from build123d import *

# Parameters (mm, degrees)
BOSS_EXTRUDE1_DEPTH = 4
SKETCH2_R           = 1.55
CUT_EXTRUDE3_DEPTH  = 130.223312929
FILLET1_R           = 5
SKETCH5_R           = 1.525
CUT_EXTRUDE4_DEPTH  = 10
SKETCH5_3_R         = 4.5
CUT_EXTRUDE5_DEPTH  = 1
CUT_EXTRUDE6_DEPTH  = 2.4
SKETCH8_W           = 140
SKETCH8_H           = 25
BOSS_EXTRUDE4_DEPTH = 5
CUT_EXTRUDE7_DEPTH  = 186.792392805
FILLET5_R           = 5
SKETCH12_W          = 5.5
SKETCH12_H          = 5
CUT_EXTRUDE8_DEPTH  = 10
FILLET6_R           = 1


with BuildPart() as part:
    # Sketch1 → Boss-Extrude1 (new body)
    with BuildSketch(Plane(origin=(0, 0, 0), x_dir=(1, 0, 0), z_dir=(0, 1, 0))):
        Polygon((-94.307015775, 45.137931034), (-94.307015775, 16.137931034), (-114.307015775, 16.137931034), (-114.307015775, 1.137931034), (-68.307015775, 1.137931034), (45.692984225, 1.137931034), (65.692984225, 1.137931034), (65.692984225, 16.137931034), (45.692984225, 16.137931034), (45.692984225, 45.137931034), (65.692984225, 45.137931034), (65.692984225, 60.137931034), (45.692984225, 60.137931034), (-68.307015775, 60.137931034), (-114.307015775, 60.137931034), (-114.307015775, 45.137931034), align=None)
    extrude(amount=BOSS_EXTRUDE1_DEPTH)

    # Sketch2 → Cut-Extrude3 (cut, through all)
    with BuildSketch(Plane(origin=(0, 4, 0), x_dir=(1, 0, 0), z_dir=(0, 1, 0))):
        with Locations(Location((40.192984225, 53.637931034, 0), (0, 0, 270))):
            Circle(SKETCH2_R)
        with Locations(Location((-69.807015775, 53.637931034, 0), (0, 0, 270))):
            Circle(SKETCH2_R)
        with Locations(Location((-69.807015775, 7.637931034, 0), (0, 0, 270))):
            Circle(SKETCH2_R)
        with Locations(Location((40.192984225, 7.637931034, 0), (0, 0, 270))):
            Circle(SKETCH2_R)
    extrude(amount=-CUT_EXTRUDE3_DEPTH, mode=Mode.SUBTRACT)

    # Fillet1
    fillet1_edges = [part.edges().sort_by_distance(p)[0] for p in [
        (65.692984225, 2, -60.137931034),
        (65.692984225, 2, -45.137931034),
        (45.692984225, 2, -45.137931034),
        (45.692984225, 2, -16.137931034),
        (65.692984225, 2, -16.137931034),
        (65.692984225, 2, -1.137931034),
        (-114.307015775, 2, -1.137931034),
        (-114.307015775, 2, -16.137931034),
        (-94.307015775, 2, -16.137931034),
        (-94.307015775, 2, -45.137931034),
        (-114.307015775, 2, -45.137931034),
        (-114.307015775, 2, -60.137931034),
    ]]
    fillet(fillet1_edges, radius=FILLET1_R)

    # Sketch5 → Cut-Extrude4 (cut)
    with BuildSketch(Plane(origin=(0, 4, 0), x_dir=(1, 0, 0), z_dir=(0, 1, 0))):
        with Locations(Location((-106.807015775, 52.637931034, 0), (0, 0, 270))):
            Circle(SKETCH5_R)
        with Locations(Location((-106.807015775, 8.637931034, 0), (0, 0, 270))):
            Circle(SKETCH5_R)
        with Locations(Location((58.192984225, 8.637931034, 0), (0, 0, 270))):
            Circle(SKETCH5_R)
        with Locations(Location((58.192984225, 52.637931034, 0), (0, 0, 270))):
            Circle(SKETCH5_R)
    extrude(amount=-CUT_EXTRUDE4_DEPTH, mode=Mode.SUBTRACT)

    # Sketch5<3> → Cut-Extrude5 (cut)
    with BuildSketch(Plane(origin=(0, 4, 0), x_dir=(1, 0, 0), z_dir=(0, 1, 0))):
        with Locations(Location((-106.807015775, 8.637931034, 0), (0, 0, 270))):
            Circle(SKETCH5_3_R)
    extrude(amount=-CUT_EXTRUDE5_DEPTH, mode=Mode.SUBTRACT)

    # Sketch6 → Cut-Extrude6 (cut)
    with BuildSketch(Plane.XZ):
        Polygon((-104.663016346, -11.019268148), (-103.672717625, -7.97184162), (-105.816717054, -5.590504507), (-108.951015204, -6.256593921), (-109.941313925, -9.304020449), (-107.797314496, -11.685357562), align=None)
        Polygon((58.770092174, -11.789826721), (61.211159934, -9.714088733), (60.634051985, -6.562193047), (57.615876277, -5.486035348), (55.174808517, -7.561773336), (55.751916465, -10.713669022), align=None)
        Polygon((60.682419613, -50.620454529), (57.690516013, -49.473278495), (55.201080626, -51.490755001), (55.703548838, -54.65540754), (58.695452437, -55.802583574), (61.184887825, -53.785107068), align=None)
        Polygon((-103.606959923, -52.473181078), (-105.349665496, -49.784226396), (-108.549721348, -49.948976352), (-110.007071626, -52.802680991), (-108.264366053, -55.491635673), (-105.064310202, -55.326885717), align=None)
    extrude(amount=-CUT_EXTRUDE6_DEPTH, mode=Mode.SUBTRACT)

    # Sketch8 → Boss-Extrude4 (add)
    with BuildSketch(Plane.XZ):
        with Locations((-24.307015775, -30.637931034)):
            Rectangle(SKETCH8_W, SKETCH8_H)
    extrude(amount=BOSS_EXTRUDE4_DEPTH)

    # Sketch9 → Cut-Extrude7 (cut, through all)
    with BuildSketch(Plane(origin=(-94.307015775, 0, -95.444946809), x_dir=(0, 0, -1), z_dir=(1, 0, 0))):
        with BuildLine():
            Line((-52.307015775, -5), (-77.307015775, -5))
            add(Edge.make_bspline(
                [(-52.307015775, -5), (-64.731276491, 0.028189696), (-77.307015775, -5)],
                knots=[0, 0, 0, 1, 1, 1], degree=2))
        make_face()
    extrude(amount=CUT_EXTRUDE7_DEPTH, mode=Mode.SUBTRACT)

    # Fillet5
    fillet5_edges = [part.edges().sort_by_distance(p)[0] for p in [
        (-24.307015775, 0, -43.137931034),
        (-24.307015775, 0, -18.137931034),
    ]]
    fillet(fillet5_edges, radius=FILLET5_R - 0.0001)  # a hair under: the kernel refuses the full size

    # Sketch12 → Cut-Extrude8 (cut)
    with BuildSketch(Plane.XZ):
        with Locations((-51.557015775, -6.637931034)):
            Rectangle(SKETCH12_W, SKETCH12_H)
        with Locations((2.942984225, -6.637931034)):
            Rectangle(SKETCH12_W, SKETCH12_H)
        with Locations((2.942984225, -54.637931034)):
            Rectangle(SKETCH12_W, SKETCH12_H)
        with Locations((-51.557015775, -54.637931034)):
            Rectangle(SKETCH12_W, SKETCH12_H)
    extrude(amount=-CUT_EXTRUDE8_DEPTH, mode=Mode.SUBTRACT)

    # Fillet6
    fillet6_edges = [part.edges().sort_by_distance(p)[0] for p in [
        (-51.557015775, 4, -9.137931034),
        (-51.557015775, 4, -4.137931034),
        (-51.557015775, 0, -9.137931034),
        (-51.557015775, 0, -4.137931034),
        (-51.557015775, 4, -52.137931034),
        (-51.557015775, 4, -57.137931034),
        (2.942984225, 4, -52.137931034),
        (2.942984225, 4, -57.137931034),
        (2.942984225, 4, -9.137931034),
        (2.942984225, 4, -4.137931034),
        (2.942984225, 0, -4.137931034),
        (2.942984225, 0, -9.137931034),
        (2.942984225, 0, -52.137931034),
        (2.942984225, 0, -57.137931034),
        (-51.557015775, 0, -57.137931034),
        (-51.557015775, 0, -52.137931034),
    ]]
    fillet(fillet6_edges, radius=FILLET6_R)


solid = part.part
Input: part model. Units: mm. Frame: model coordinates. A direction names the side the tool comes from. Coordinates: 2 decimals unless noted, no trailing zeros.
(1) Pull-direction query (Z, two-part tool) for faces 5 (the face through (-112.8, 2.03, -46.56)), 6 (the face through (65.693, 2, -9)), 7 (the face through (0.193, 2, -55)), 8 (the face through (-112.881, 2.028, -58.634)); classes: released by +Z, released by -Z, zero draft, split by the parting line, or undercut.
(2) Set-up query: faces 1 (the face through (-95.733, 2.028, -17.641)), 2 (the face through (-109, 3, -9)), 3 (the face through (64.267, 2.028, -46.641)), 4 (the face through (-105, 2.4, -52)). Return all of +Z, -Z, +X, -X, +Y, -Y with unobstructed straight access to the full face (end or side cutting, diameter ignored); none if empty.
(3) First-contact query: pin 1 Ø5 at (y, z) = (-0.5, -33) entering from +X; pin 2 Ø1 at (x, z) = (-17, -19.5) entering from -Y; pin 3 Ø11.5 at (x, z) = (-106.81, -8.64) entering from -Y; pin 4 Ø2.5 at (x, z) = (-106.81, -8.64) entering from +Y. Flat tips, straight axial feed; report the tip coordinate or a pass-through.
(4) Material intervals for probe 1 along X at (y, z) = (3, -55.5); probe 2 along X at (y, z) = (-1, -37.5); probe 3 along Y at (x, z) = (-63.5, -31), sorted ascending.
Data:
1. face 5: undercut
1. face 6: zero draft
1. face 7: undercut
1. face 8: released by -Z
2. face 1: -X, +Y, -Y
2. face 2: +Y
2. face 3: +X, +Y, -Y
2. face 4: -Y
3. pin 1: stops at x = 45.69
3. pin 2: stops at y = -4.67
3. pin 3: stops at y = 0
3. pin 4: passes through
4. probe 1: x = -114.29 to -54.31, -48.81 to 0.19, 5.69 to 65.68
4. probe 2: x = -94.31 to 45.69
4. probe 3: y = -2.49 to 4
